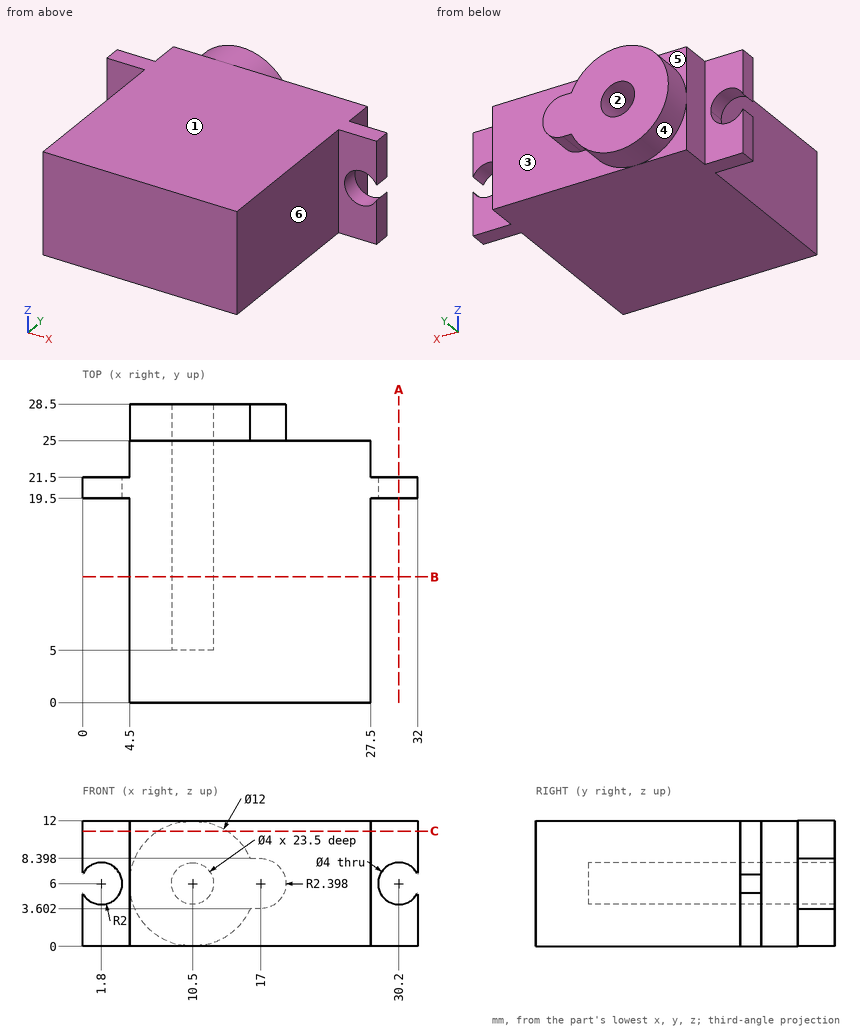
Print and shaded views of the part. All mm, measured from the part's lowest x, y and z. A direction names the side the tool comes from. Coordinates: 2 decimals unless noted, no trailing zeros. Loops run counter-clockwise (first coordinate to the right, second up) from the corner with the lowest first, then second, coordinate; pieces in that order, holes last. Notation, with made-up numbers: M 60.25,10 L 111.25,10 A24 cw 111.25,21 Z; hole C -12.75,-27 d10. An arc over 180 degrees is marked long. Use a Markdown table: item, result. Add a question column.
Q1. Which spindle directions (+Z, -Z, +X, -X, +Y, -Y) get a long thin tool onto all of the face, cutting with end or side? Do the marked faces 4, 5 and 6. Say none if no direction does.
Q2. Probe L1, parallel to X at y = 20.8, z = 6; L2, parallel to Z at x = 30.2, y = 20.3; L3, parallel to X at y = 13.5, z = 6. List the from-to ranges inside material, lowest first.
Q3. Mould opens along Z. For the marked faces 1, 2 and 3 say: +Z half, -Z half, draft (parallel to the pull), parting line (faces both ways), or undercut.
Q4. Pin check, flat tips, straight feed: P1, Ø1, axis at y = 24, z = 3.5, coming from the +X side; P2, Ø4, axis at y = 14, z = 2, coming from the -X side; P3, Ø2, axis at x = 31, z = 3.5, coming from the -Y side; P4, Ø1.3, axis at x = 1.5, z = 7, coming from the +Y side. Stop position of each tip, or through.
Q5. Cut at B-B (y = 12). Write the cut outline in (x, z).
Q6. Cut at C-C (z = 11). Write the cut outline in (x, y).
Q7. Cut at A-A (x = 30.2). Write the cut outline in (y, z).
Worked out:
| question | item | result |
|---|---|---|
| 1 | face 4 | +Y |
| 1 | face 5 | +Z, -X, +Y |
| 1 | face 6 | +Z, -Z, +X, -Y |
| 2 | L1 | x = 3.8 to 8.5, 12.5 to 28.2 |
| 2 | L2 | z = 0 to 4, 8 to 12 |
| 2 | L3 | x = 4.5 to 8.5, 12.5 to 27.5 |
| 3 | face 1 | +Z half |
| 3 | face 2 | undercut |
| 3 | face 3 | draft |
| 4 | P1 | stops at x = 27.5 |
| 4 | P2 | stops at x = 4.5 |
| 4 | P3 | stops at y = 19.5 |
| 4 | P4 | passes through |
| 5 | outline | M 4.5,0 L 27.5,0 L 27.5,12 L 4.5,12 Z; hole C 10.5,6 d4 |
| 6 | outline | M 0,19.5 L 4.5,19.5 L 4.5,0 L 27.5,0 L 27.5,19.5 L 32,19.5 L 32,21.5 L 27.5,21.5 L 27.5,25 L 13.82,25 L 13.82,28.5 L 7.18,28.5 L 7.18,25 L 4.5,25 L 4.5,21.5 L 0,21.5 Z |
| 7 | outline | M 19.5,0 L 21.5,0 L 21.5,4 L 19.5,4 Z; M 19.5,8 L 21.5,8 L 21.5,12 L 19.5,12 Z |
